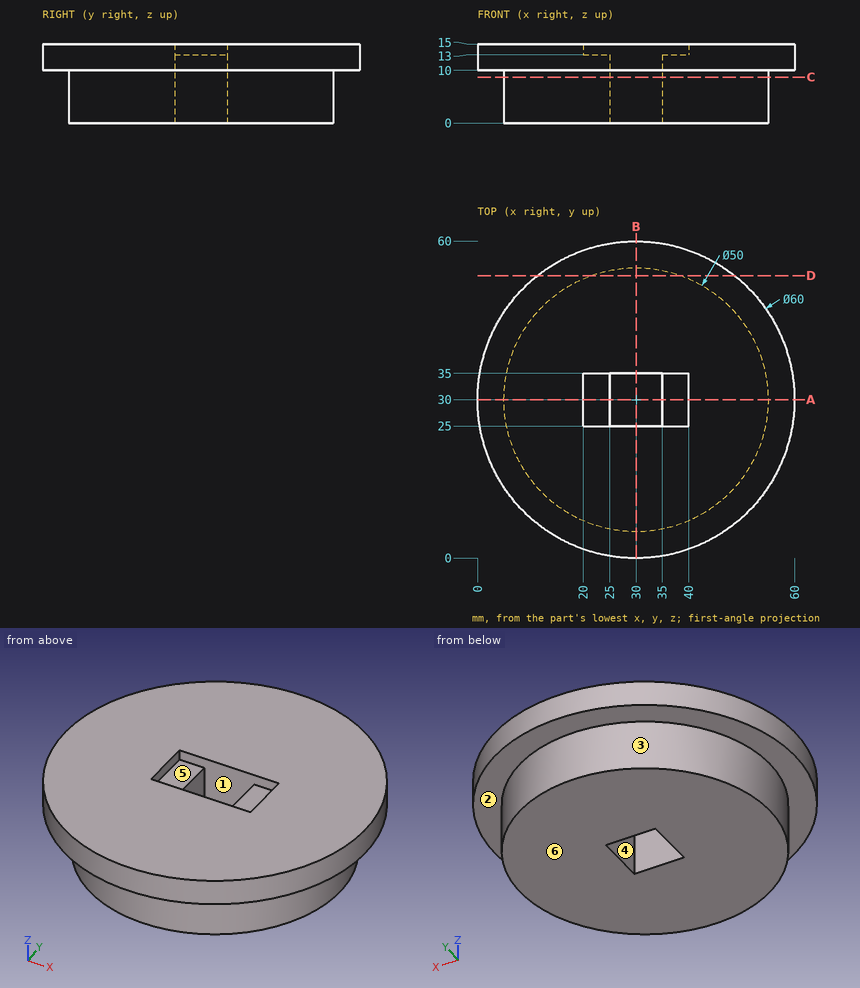
Verification items for this drawing (mm, ordinates from the low corner). A direction names the side the tool comes from. Coordinates: 2 decimals unless noted, no trailing zeros. Loops run counter-clockwise (first coordinate to the right, second up) from the corner with the lowest first, then second, coordinate; pieces in that order, holes last. Notation, with made-up numbers: (53, 33) -> (71, 33) arc R27 cw to (71, 52) -> close; hole circle Ø8 at (-1, 11.25). An arc over 180 degrees is marked (long way). Put each result on its own line as item: value.
1. Tool access check on the marked faces 5 and 6. Record the directions out of +Z, -Z, +X, -X, +Y, -Y that give a thin tool (end or side, any length) a straight path to the whole face; none if there is none.
Result set:
face 5: +Z
face 6: -Z, +X, -X, +Y, -Y
2. Gauge pin test, flat ends, axial feed: P1, Ø8, axis at y = 28, z = 8.5, coming from the -X side; P2, Ø8, axis at y = 31.5, z = 3, coming from the -X side; P3, Ø7.5, axis at x = 30.5, z = 8.5, coming from the -Y side; P4, Ø0.6, axis at y = 28, z = 14.5, coming from the +X side. Record the tip position at first contact, or that the pin passes through.
Result set:
P1: stops at x = 0
P2: stops at x = 5
P3: stops at y = 0
P4: stops at x = 59.95
3. Section check B-B, the plane x = 30. Record the boundary of the cut face in (y, z).
Result set:
outline: (0, 10) -> (5, 10) -> (5, 0) -> (25, 0) -> (25, 15) -> (0, 15) -> close; (35, 0) -> (55, 0) -> (55, 10) -> (60, 10) -> (60, 15) -> (35, 15) -> close
4. Thickness scan on line 1 (Z direction, x = 45, y = 53.5); line 2 (Y direction, x = 27.5, z = 8.5); line 3 (Z direction, x = 35.5, y = 27). Record the ranges inside material, lowest first.
Result set:
line 1: z = 10 to 15
line 2: y = 5.13 to 25, 35 to 54.87
line 3: z = 0 to 13
5. Section check C-C, the plane z = 8.75. Record the boundary of the cut face in (x, y), then the cut area to 3 significant figures.
Result set:
outline: circle Ø50 at (30, 30); hole (25, 25) -> (35, 25) -> (35, 35) -> (25, 35) -> close
area: 1,860 mm^2
6. Mould release check, pull along Y, two halves, no side actions. Record for the marked faces 1, 2, 3 and 4: pulls with the +Y half, pulls with the -Y half, needs draft (parallel to the pull), parting line crosses it, or undercut.
Result set:
face 1: undercut
face 2: needs draft
face 3: parting line crosses it
face 4: undercut
7. Section check A-A, the plane y = 30. Record the boundary of the cut face in (x, z), then the cut area to 3 significant figures.
Result set:
outline: (0, 10) -> (5, 10) -> (5, 0) -> (25, 0) -> (25, 13) -> (20, 13) -> (20, 15) -> (0, 15) -> close; (35, 0) -> (55, 0) -> (55, 10) -> (60, 10) -> (60, 15) -> (40, 15) -> (40, 13) -> (35, 13) -> close
area: 630 mm^2
8. Section check D-D, the plane y = 53.5. Record the boundary of the cut face in (x, z), then the cut area to 3 significant figures.
Result set:
outline: (11.35, 10) -> (21.47, 10) -> (21.47, 0) -> (38.53, 0) -> (38.53, 10) -> (48.65, 10) -> (48.65, 15) -> (11.35, 15) -> close
area: 357 mm^2
